from build123d import *

# Parameters (mm, degrees)
SKETCH_1_W                  = 710
SKETCH_1_H                  = 300
EXTRUDE_1_DEPTH             = 11.5
SKETCH_2_R                  = 13
CUT_EXTRUDE_1_DEPTH         = 386.560954973
PATTERN_LINEAR_1_COUNT      = 4
PATTERN_LINEAR_1_PITCH      = 80
PATTERN_LINEAR_1_COUNT_DIR2 = 3
PATTERN_LINEAR_1_PITCH_DIR2 = 80
SKETCH_3_W                  = 710
SKETCH_3_H                  = 11.5
EXTRUDE_2_DEPTH             = 89


with BuildPart() as part:
    # 草图1 → 凸台-拉伸1 (new body)
    with BuildSketch(Plane.XY):
        Rectangle(SKETCH_1_W, SKETCH_1_H)
    extrude(amount=EXTRUDE_1_DEPTH)

    # 草图2 → 切除-拉伸1 (cut, through all)
    with BuildSketch(Plane.XY.offset(11.5)):
        with Locations((-300, 80)):
            Circle(SKETCH_2_R)
        with Locations((60, 80)):
            Circle(SKETCH_2_R)
    cut_extrude_1 = extrude(amount=-CUT_EXTRUDE_1_DEPTH, mode=Mode.SUBTRACT)

    # 阵列(线性)1: Cut-Extrude 1 4 × 3
    with Locations(*[(i * PATTERN_LINEAR_1_PITCH, -j * PATTERN_LINEAR_1_PITCH_DIR2, 0) for i in range(PATTERN_LINEAR_1_COUNT) for j in range(PATTERN_LINEAR_1_COUNT_DIR2) if (i, j) != (0, 0)]):
        add(cut_extrude_1, mode=Mode.SUBTRACT)

    # 草图3 → 凸台-拉伸2 (add)
    with BuildSketch(Plane.XY.offset(11.5)):
        with Locations((0, 144.25)):
            Rectangle(SKETCH_3_W, SKETCH_3_H)
    extrude_2 = extrude(amount=EXTRUDE_2_DEPTH)

    # 镜向1: 凸台-拉伸2 across plane
    add(extrude_2.mirror(Plane.ZX))


solid = part.part
Source: CAD feature listing. Evaluate the final solid. Frame: model axes, mm. A direction names the side the tool comes from. Give positions to 0.01 mm unless a question says otherwise; leave off trailing zeros. Order: outer loops, then holes, each group sorted by start corner. A loop starts at its lowest first (then second) coordinate and runs counter-clockwise, first axis right, second up. Notation, with made-up numbers: (-4, 85.25) -> (5, 85.25) arc R14 ccw to (5, 108.25) -> close; hole circle Ø7 at (-34.5, 75.25). An arc over 180 degrees is marked (long way). Write item = value, one per line.
Item 1: Set-up query: faces 4 (the face through (-5, -138.5, 55)), 5 (the face through (-70.316, -7.91, 5.83)). Return all of +Z, -Z, +X, -X, +Y, -Y with unobstructed straight access to the full face (end or side cutting, diameter ignored); none if empty.
Check result:
face_4 = +Z, +X, -X
face_5 = +Z, -Z
Item 2: Mould query, pull axis X, two halves, no side actions, for faces 1 (the face through (355, 1, 9)), 2 (the face through (-232.987, -79.428, 5.83)), 3 (the face through (-5, 138.5, 55)). Classes: +X half, -X half, draft (parallel to the pull), parting line (faces both ways), or undercut.
Check result:
face_1 = +X half
face_2 = undercut
face_3 = draft
Item 3: Section query C-C (y = 80). State how many separate pieces and enclosed holes the cut face has, then the cut area to 3 significant figures.
Check result:
separate_pieces = 9
enclosed_holes = 0
area = 5,770 mm²
Item 4: Section query A-A (x = -60). Output: boundary loops of the cut face in (y, z), then the cut area to 3 significant figures.
Check result:
outline = (-150, 0) -> (-93, 0) -> (-93, 11.5) -> (-138.5, 11.5) -> (-138.5, 100.5) -> (-150, 100.5) -> close; (-67, 0) -> (-13, 0) -> (-13, 11.5) -> (-67, 11.5) -> close; (13, 0) -> (67, 0) -> (67, 11.5) -> (13, 11.5) -> close; (93, 0) -> (150, 0) -> (150, 100.5) -> (138.5, 100.5) -> (138.5, 11.5) -> (93, 11.5) -> close
area = 4,600 mm²
Item 5: Ray query, probe 1 along Y at (x, z) = (140, 8); probe 2 along Y at (x, z) = (93, 73.5); probe 3 along Z at (x, y) = (21, -47). Return the intervals inside material, ascending.
Check result:
probe_1 = -150 to -93, -67 to -13, 13 to 67, 93 to 150
probe_2 = -150 to -138.5, 138.5 to 150
probe_3 = 0 to 11.5
Item 6: Contact query for flat-ended pins moving along their axis: pin 1 (15.5 mm diameter, centred on x = 60, y = 0, fed in from -Z); pin 2 (12 mm diameter, centred on x = -61.5, y = 49, fed in from +Z). Output: stop coordinate, or through.
Check result:
pin_1 = through
pin_2 = 11.5
Item 7: Section query B-B (z = 81.5). Output: boundary loops of the cut face in (x, y).
Check result:
outline = (-355, -150) -> (355, -150) -> (355, -138.5) -> (-355, -138.5) -> close; (-355, 138.5) -> (355, 138.5) -> (355, 150) -> (-355, 150) -> close
Item 8: Section query D-D (x = -183). Output: boundary loops of the cut face in (y, z).
Check result:
outline = (-150, 0) -> (150, 0) -> (150, 100.5) -> (138.5, 100.5) -> (138.5, 11.5) -> (-138.5, 11.5) -> (-138.5, 100.5) -> (-150, 100.5) -> close
